from build123d import *

# Parameters (mm, degrees)
BOX022_W     = 1168.4
BOX022_H     = 558.8
BOX022_DEPTH = 457.2
BOX021_W     = 1168.4
BOX021_H     = 558.8
BOX021_DEPTH = 457.2
BOX020_W     = 1168.4
BOX020_H     = 558.8
BOX020_DEPTH = 457.2
BOX019_W     = 1168.4
BOX019_H     = 558.8
BOX019_DEPTH = 457.2
BOX018_W     = 1219.2
BOX018_H     = 609.6
BOX018_DEPTH = 2133.6


with BuildPart() as cube022:
    # Box022 → Box022 (new body)
    with BuildSketch(Plane(origin=(25.4, 0, 1651), x_dir=(1, 0, 0), z_dir=(0, 0, 1))):
        with Locations((584.2, 279.4)):
            Rectangle(BOX022_W, BOX022_H)
    extrude(amount=BOX022_DEPTH)


with BuildPart() as cube021:
    # Box021 → Box021 (new body)
    with BuildSketch(Plane(origin=(25.4, 0, 685.8), x_dir=(1, 0, 0), z_dir=(0, 0, 1))):
        with Locations((584.2, 279.4)):
            Rectangle(BOX021_W, BOX021_H)
    extrude(amount=BOX021_DEPTH)


with BuildPart() as cube020:
    # Box020 → Box020 (new body)
    with BuildSketch(Plane(origin=(25.4, 0, 203.2), x_dir=(1, 0, 0), z_dir=(0, 0, 1))):
        with Locations((584.2, 279.4)):
            Rectangle(BOX020_W, BOX020_H)
    extrude(amount=BOX020_DEPTH)


with BuildPart() as cube019:
    # Box019 → Box019 (new body)
    with BuildSketch(Plane(origin=(25.4, 0, 1168.4), x_dir=(1, 0, 0), z_dir=(0, 0, 1))):
        with Locations((584.2, 279.4)):
            Rectangle(BOX019_W, BOX019_H)
    extrude(amount=BOX019_DEPTH)


with BuildPart() as cut009:
    # Box018 → Box018 (new body)
    with BuildSketch(Plane.XY):
        with Locations((609.6, 304.8)):
            Rectangle(BOX018_W, BOX018_H)
    extrude(amount=BOX018_DEPTH)

    # Cut006: cut Cube019
    add(cube019.part, mode=Mode.SUBTRACT)

    # Cut007: cut Cube020
    add(cube020.part, mode=Mode.SUBTRACT)

    # Cut008: cut Cube021
    add(cube021.part, mode=Mode.SUBTRACT)

    # Cut009: cut Cube022
    add(cube022.part, mode=Mode.SUBTRACT)


with BuildPart() as cut009_1:
    # Cut009 placement: moved
    add(cut009.part.moved(Location((3792, 4261, 0))))


solid = cut009_1.part
Part model, mm, in its own coordinate system. A direction names the side the tool comes from. Give positions to 0.01 mm unless a question says otherwise; leave off trailing zeros. Loops run counter-clockwise (first coordinate to the right, second up) from the corner with the lowest first, then second, coordinate; pieces in that order, holes last.
(1) Drill centre lines: line 1 along Z through (x, y) = (4648, 4346); line 2 along X through (y, z) = (4633, 1664.5); line 3 along Y through (x, z) = (4529, 1907.5). Where is each one in solid material? Low to high.
Return value:
line 1: z = 0 to 203.2, 660.4 to 685.8, 1143 to 1168.4, 1625.6 to 1651, 2108.2 to 2133.6
line 2: x = 3792 to 3817.4, 4985.8 to 5011.2
line 3: y = 4819.8 to 4870.6
(2) Band-saw the part on B-B (y = 4590.5). Write the cut outline in (x, z), and give its area (3 significant figures).
Return value:
outline: (3792, 0) - (5011.2, 0) - (5011.2, 2133.6) - (3792, 2133.6) - close; hole (3817.4, 203.2) - (4985.8, 203.2) - (4985.8, 660.4) - (3817.4, 660.4) - close; hole (3817.4, 685.8) - (4985.8, 685.8) - (4985.8, 1143) - (3817.4, 1143) - close; hole (3817.4, 1168.4) - (4985.8, 1168.4) - (4985.8, 1625.6) - (3817.4, 1625.6) - close; hole (3817.4, 1651) - (4985.8, 1651) - (4985.8, 2108.2) - (3817.4, 2108.2) - close
area: 465,000 mm2
(3) Band-saw the part on C-C (z = 1529.5). Write the cut outline in (x, y).
Return value:
outline: (3792, 4261) - (3817.4, 4261) - (3817.4, 4819.8) - (4985.8, 4819.8) - (4985.8, 4261) - (5011.2, 4261) - (5011.2, 4870.6) - (3792, 4870.6) - close
(4) Band-saw the part on A-A (x = 4760). Write the cut outline in (y, z), and give its area (3 significant figures).
Return value:
outline: (4261, 0) - (4870.6, 0) - (4870.6, 2133.6) - (4261, 2133.6) - (4261, 2108.2) - (4819.8, 2108.2) - (4819.8, 1651) - (4261, 1651) - (4261, 1625.6) - (4819.8, 1625.6) - (4819.8, 1168.4) - (4261, 1168.4) - (4261, 1143) - (4819.8, 1143) - (4819.8, 685.8) - (4261, 685.8) - (4261, 660.4) - (4819.8, 660.4) - (4819.8, 203.2) - (4261, 203.2) - close
area: 279,000 mm2
(5) Pull direction X, two halves, no side cores. Call faces 1 (the flat face through (4393, 4570, 2133.6)), 2 (the flat face through (4393, 4544, 1143)), 3 (the flat face through (5011.2, 4562, 1052)): pulls with the +X half, pulls with the -X half, needs draft (parallel to the pull), parting line crosses it, or undercut.
Return value:
face 1: needs draft
face 2: undercut
face 3: pulls with the +X half
(6) Pin check, flat tip, straight feed: pin 1 (2 mm diameter, centred on x = 4017.5, z = 843.5, fed in from -Y). Stop position of the tip, or through.
Return value:
pin 1: stops at y = 4819.8
(7) 3-axis set-ups, long thin cutter, end or side, ignore diameter. For faces 4 (the flat face through (4393, 4819.8, 429)), 5 (the flat face through (3792, 4562, 1052)): which of +Z, -Z, +X, -X, +Y, -Y reach the whole face in a straight line?
Return value:
face 4: -Y
face 5: +Z, -Z, -X, +Y, -Y
